from build123d import *

# Parameters (mm, degrees)
SKETCH3_W           = 159
SKETCH3_H           = 300
BOSS_EXTRUDE1_DEPTH = 10
SKETCH4_W           = 10
SKETCH4_H           = 10
BOSS_EXTRUDE2_DEPTH = 50
SKETCH7_R           = 2
SKETCH7_R_2         = 2.000000006
SKETCH7_R_3         = 1.999999994
CUT_EXTRUDE2_DEPTH  = 10


with BuildPart() as part:
    # Sketch3 → Boss-Extrude1 (new body)
    with BuildSketch(Plane(origin=(0, 0, 0), x_dir=(1, 0, 0), z_dir=(0, 1, 0))):
        Rectangle(SKETCH3_W, SKETCH3_H)
    extrude(amount=BOSS_EXTRUDE1_DEPTH)

    # Sketch4 → Boss-Extrude2 (add)
    with BuildSketch(Plane(origin=(0, 10, 0), x_dir=(1, 0, 0), z_dir=(0, 1, 0))):
        with Locations((74.5, -145)):
            Rectangle(SKETCH4_W, SKETCH4_H)
        with Locations((74.5, -80)):
            Rectangle(SKETCH4_W, SKETCH4_H)
        with Locations((9.5, -145)):
            Rectangle(SKETCH4_W, SKETCH4_H)
        with Locations((9.5, -80)):
            Rectangle(SKETCH4_W, SKETCH4_H)
    extrude(amount=BOSS_EXTRUDE2_DEPTH)

    # Sketch7 → Cut-Extrude2 (cut)
    with BuildSketch(Plane.XZ):
        with Locations(Location((34.5, -105, 0), (0, 0, 270))):
            Circle(SKETCH7_R)
        with Locations(Location((72.5, -105, 0), (0, 0, 270))):
            Circle(SKETCH7_R)
        with Locations(Location((72.5, -65, 0), (0, 0, 270))):
            Circle(SKETCH7_R)
        with Locations(Location((34.5, -65, 0), (0, 0, 270))):
            Circle(SKETCH7_R)
        with Locations(Location((-34.5, -65, 0), (0, 0, 270))):
            Circle(SKETCH7_R)
        with Locations(Location((-72.5, -65, 0), (0, 0, 270))):
            Circle(SKETCH7_R)
        with Locations(Location((-34.5, -105, 0), (0, 0, 270))):
            Circle(SKETCH7_R)
        with Locations(Location((-72.5, -105, 0), (0, 0, 270))):
            Circle(SKETCH7_R)
        with Locations(Location((-72.5, 65, 0), (0, 0, 270))):
            Circle(SKETCH7_R)
        with Locations(Location((-72.5, 105, 0), (0, 0, 270))):
            Circle(SKETCH7_R)
        with Locations(Location((-34.5, 105, 0), (0, 0, 270))):
            Circle(SKETCH7_R_2)
        with Locations(Location((-34.5, 65, 0), (0, 0, 270))):
            Circle(SKETCH7_R)
        with Locations(Location((34.5, 105, 0), (0, 0, 270))):
            Circle(SKETCH7_R_3)
        with Locations(Location((72.5, 105, 0), (0, 0, 270))):
            Circle(SKETCH7_R)
        with Locations(Location((72.5, 65, 0), (0, 0, 270))):
            Circle(SKETCH7_R)
        with Locations(Location((34.5, 65, 0), (0, 0, 270))):
            Circle(SKETCH7_R)
    extrude(amount=-CUT_EXTRUDE2_DEPTH, mode=Mode.SUBTRACT)


solid = part.part
Can you work these out from the model? Positions are in its coordinate system, mm. A direction names the side the tool comes from. Coordinates: 2 decimals unless noted, no trailing zeros. Loops run counter-clockwise (first coordinate to the right, second up) from the corner with the lowest first, then second, coordinate; pieces in that order, holes last. Notation, with made-up numbers: (87, -8) - (110, -8) arc R13 ccw to (110, 1) - close; hole circle Ø2 at (52, 83). An arc over 180 degrees is marked (long way). Put each result on its own line as item: value. Start each with the question number.
Item 1: For pin 1 (5 mm diameter, centred on y = 27.5, z = 78.5, fed in from -X); pin 2 (4.5 mm diameter, centred on x = 72.5, z = 105, fed in from +Y); pin 3 (3 mm diameter, centred on x = 74.5, y = 28, fed in from -Z), each with a flat end and sliding along its axis, tell me the tip position at first contact or that it passes through.
Item 2: Suppose I cut it at B-B (x = 10.5). Please give me the cut outline in (y, z).
Item 3: Suppose I cut it at A-A (y = 53.5). Please give me the cut outline in (x, z).
Item 4: Which directions (+Z, -Z, +X, -X, +Y, -Y) give clear straight access to the entire face, cutting with the end or side of a thin tool? Please do faces 1 (the face through (74, 35, 85)), 2 (the face through (14.5, 35, 145)), 3 (the face through (4.5, 35, 145)).
Item 5: If we mould it in two halves opening along Z, with no side actions, what happens to faces 4 (the face through (79.5, 8, 23)), 5 (the face through (74, 35, 140)), 6 (the face through (11, 14, 150))? For each: +Z half, -Z half, draft (parallel to the pull), parting line (faces both ways), or undercut.
Item 6: If I drill on line 1 along X through (y, z) = (3, -65); line 2 along Y through (x, z) = (16.5, -25); line 3 along X through (y, z) = (48, 84), over which ranges is the centre line in solid material (lowest first)?
Item 7: Suppose I cut it at C-C (z = 3). Please give me the cut outline in (x, y).
Item 8: Suppose I cut it at D-D (x = -58). Please give me the cut outline in (y, z).
Here are the results:
1. pin 1: x = 4.5
1. pin 2: y = 10
1. pin 3: z = 75
2. outline: (0, -150) - (10, -150) - (10, 75) - (60, 75) - (60, 85) - (10, 85) - (10, 140) - (60, 140) - (60, 150) - (0, 150) - close
3. outline: (4.5, 75) - (14.5, 75) - (14.5, 85) - (4.5, 85) - close; (4.5, 140) - (14.5, 140) - (14.5, 150) - (4.5, 150) - close; (69.5, 75) - (79.5, 75) - (79.5, 85) - (69.5, 85) - close; (69.5, 140) - (79.5, 140) - (79.5, 150) - (69.5, 150) - close
4. face 1: +X, -X, +Y
4. face 2: +Z, -Z, +Y
4. face 3: +Z, -Z, -X, +Y
5. face 4: draft
5. face 5: undercut
5. face 6: +Z half
6. line 1: -79.5 to -74.5, -70.5 to -36.5, -32.5 to 32.5, 36.5 to 70.5, 74.5 to 79.5
6. line 2: 0 to 10
6. line 3: 4.5 to 14.5, 69.5 to 79.5
7. outline: (-79.5, 0) - (79.5, 0) - (79.5, 10) - (-79.5, 10) - close
8. outline: (0, -150) - (10, -150) - (10, 150) - (0, 150) - close
